Verification items for this drawing (mm, ordinates from the low corner). A direction names the side the tool comes from. Coordinates: 2 decimals unless noted, no trailing zeros. Order: outer loops, then holes, each group sorted by start corner. A loop starts at its lowest first (then second) coordinate and runs counter-clockwise, first axis right, second up. Notation, with made-up numbers: (68, 40.25) -> (127, 40.25) arc R19 cw to (127, 46.25) -> close; hole circle Ø11 at (17.5, 43.5). An arc over 180 degrees is marked (long way). Answer in a Markdown table with one row per item. Add a question column.
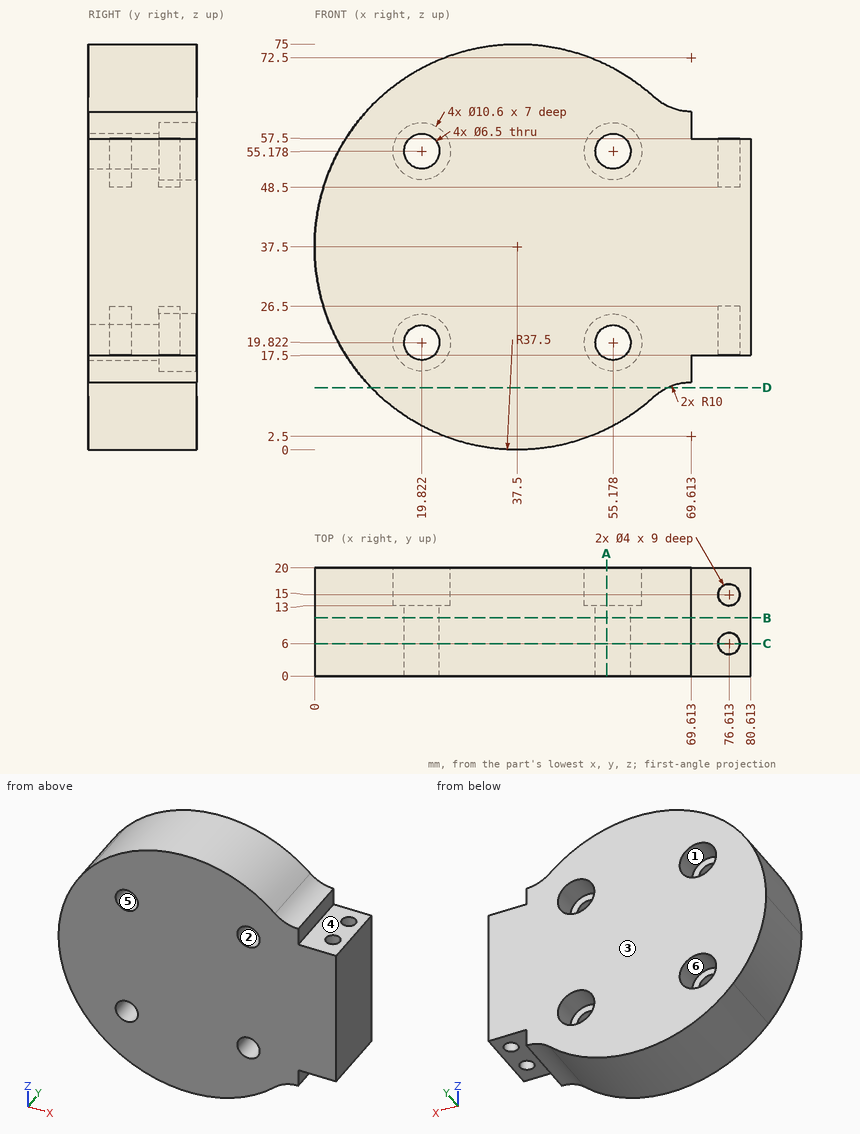
(1) Go/stop test with flat-tipped pins: P1, Ø5.5, axis at x = 20.5, z = 57.5, coming from the +Y side; P2, Ø12, axis at y = 17, z = 47.5, coming from the -X side; P3, Ø5, axis at x = 76.61, y = 6, coming from the -Z side. Record where each tip stops, or that it passes through.
(2) Cross-section at C-C (y = 6). Enter the section's corners in (x, z).
(3) Cross-section at D-D (z = 11.5). Enter the section's corners in (x, y), plus the area to 3 significant figures.
(4) Cross-section at A-A (x = 54). Enter the section's corners in (y, z) (1 decimal), plus the area to 3 significant figures.
(5) Scan lines: line 1 along Z through (x, y) = (56, 7.75); line 2 along X through (y, z) = (7.5, 18.5) (1 decimal); line 3 along Z through (x, y) = (21, 5.75) (1 decimal). Record each from-to range of solid material in increasing order.
(6) Mould release check, pull along Z, two halves, no side actions. Record for the marked faces 1, 2, 3 and 4: +Z half, -Z half, draft (parallel to the pull), parting line (faces both ways), or undercut.
(7) Cross-section at B-B (y = 10.75). Enter the section's corners in (x, z), plus the area to 3 significant figures.
(8) Access from +Z, -Z, +X, -X, +Y, -Y to the whole of each face (thin tool, end or side, straight path). Record for the marked faces 5 and 6.
Checks:
| question | item | result |
|---|---|---|
| 1 | P1 | y = 13 |
| 1 | P2 | x = 0.21 |
| 1 | P3 | z = 17.5 |
| 2 | outline | (62.85, 9.87) arc R10 cw to (69.61, 12.5) -> (69.61, 17.5) -> (74.61, 17.5) -> (74.61, 26.5) -> (78.61, 26.5) -> (78.61, 17.5) -> (80.61, 17.5) -> (80.61, 57.5) -> (78.61, 57.5) -> (78.61, 48.5) -> (74.61, 48.5) -> (74.61, 57.5) -> (69.61, 57.5) -> (69.61, 62.5) arc R10 cw to (62.85, 65.13) arc R37.5 ccw (long way) to start; hole circle Ø6.5 at (19.82, 19.82); hole circle Ø6.5 at (19.82, 55.18); hole circle Ø6.5 at (55.18, 19.82); hole circle Ø6.5 at (55.18, 55.18) |
| 3 | outline | (10.48, 0) -> (65.25, 0) -> (65.25, 20) -> (10.48, 20) -> close |
| 3 | area | 1,100 mm² |
| 4 | outline | (0, 3.8) -> (20, 3.8) -> (20, 14.7) -> (13, 14.7) -> (13, 16.8) -> (0, 16.8) -> close; (0, 22.9) -> (13, 22.9) -> (13, 25) -> (20, 25) -> (20, 50) -> (13, 50) -> (13, 52.1) -> (0, 52.1) -> close; (0, 58.2) -> (13, 58.2) -> (13, 60.3) -> (20, 60.3) -> (20, 71.2) -> (0, 71.2) -> close |
| 4 | area | 1,040 mm² |
| 5 | line 1 | 4.88 to 16.68, 22.97 to 52.03, 58.32 to 70.12 |
| 5 | line 2 | 5.2 to 16.9, 22.8 to 52.2, 58.1 to 75.3, 77.9 to 80.6 |
| 5 | line 3 | 3.8 to 16.8, 22.9 to 52.1, 58.2 to 71.2 |
| 6 | face 1 | undercut |
| 6 | face 2 | undercut |
| 6 | face 3 | draft |
| 6 | face 4 | +Z half |
| 7 | outline | (62.85, 9.87) arc R10 cw to (69.61, 12.5) -> (69.61, 17.5) -> (80.61, 17.5) -> (80.61, 57.5) -> (69.61, 57.5) -> (69.61, 62.5) arc R10 cw to (62.85, 65.13) arc R37.5 ccw (long way) to start; hole circle Ø6.5 at (19.82, 19.82); hole circle Ø6.5 at (19.82, 55.18); hole circle Ø6.5 at (55.18, 19.82); hole circle Ø6.5 at (55.18, 55.18) |
| 7 | area | 4,610 mm² |
| 8 | face 5 | +Y, -Y |
| 8 | face 6 | +Y |
